```python
from build123d import *

# Parameters (mm, degrees)
BOSS_EXTRUDE1_DEPTH      = 1
SKETCH2_W                = 5
SKETCH2_H                = 4
BOSS_EXTRUDE2_DEPTH      = 1.5
CHAMFER1_SIZE            = 0.25
SKETCH4_W                = 0.5
SKETCH4_H                = 1
BOSS_EXTRUDE3_DEPTH      = 0.5
BOSS_EXTRUDE4_DEPTH      = 0.4
CHAMFER1_OF_MIRROR1_SIZE = 0.25
SKETCH6_R                = 4
BOSS_EXTRUDE5_DEPTH      = 1.5
SKETCH7_W                = 3
SKETCH7_H                = 1
BOSS_EXTRUDE6_DEPTH      = 2
BOSS_EXTRUDE7_DEPTH      = 3
CUT_EXTRUDE1_DEPTH       = 3
SKETCH10_R               = 2.5
BOSS_EXTRUDE8_DEPTH      = 0.25
CUT_EXTRUDE2_DEPTH       = 0.25
SKETCH13_R               = 2.5
BOSS_EXTRUDE11_DEPTH     = 0.25
BOSS_EXTRUDE12_START     = -0.25
SKETCH14_R               = 2.5
BOSS_EXTRUDE12_DEPTH     = 0.25
SKETCH15_R               = 3.75
BOSS_EXTRUDE13_DEPTH     = 2.5
SKETCH17_R               = 0.75
CUT_EXTRUDE3_DEPTH       = 3
CUT_EXTRUDE5_DEPTH       = 7


with BuildPart() as part:
    # Sketch1 → Boss-Extrude1 (new body)
    with BuildSketch(Plane(origin=(0, 0, 0), x_dir=(1, 0, 0), z_dir=(0, 1, 0))):
        with BuildLine():
            Line((8.75, -5), (-7.25, -5))
            ThreePointArc((-7.25, -5), (-7.689339828, -3.939339828), (-8.75, -3.5))
            Line((-8.75, -3.5), (-8.75, 3.5))
            ThreePointArc((-8.75, 3.5), (-7.689339828, 3.939339828), (-7.25, 5))
            Line((-7.25, 5), (8.75, 5))
            Line((8.75, 5), (8.75, -5))
        make_face()
    extrude(amount=BOSS_EXTRUDE1_DEPTH)

    # Sketch2 → Boss-Extrude2 (add)
    with BuildSketch(Plane(origin=(0, 1, 0), x_dir=(1, 0, 0), z_dir=(0, 1, 0))):
        with Locations((4.283897802, -1)):
            Rectangle(SKETCH2_W, SKETCH2_H)
    boss_extrude2 = extrude(amount=BOSS_EXTRUDE2_DEPTH)

    # Chamfer1
    chamfer1_edges = [part.edges().sort_by_distance(p)[0] for p in [
        (6.783897802, 2.5, 1),
        (4.283897802, 2.5, -1),
        (1.783897802, 2.5, 1),
        (4.283897802, 2.5, 3),
    ]]
    chamfer(chamfer1_edges, length=CHAMFER1_SIZE)

    # Sketch4 → Boss-Extrude3 (add)
    with BuildSketch(Plane(origin=(0, 1, 0), x_dir=(1, 0, 0), z_dir=(0, 1, 0))):
        with Locations((5.033897802, -3.5)):
            Rectangle(SKETCH4_W, SKETCH4_H)
        with Locations((6.533897802, -3.5)):
            Rectangle(SKETCH4_W, SKETCH4_H)
        with Locations((3.533897802, -3.5)):
            Rectangle(SKETCH4_W, SKETCH4_H)
        with Locations((2.033897802, -3.5)):
            Rectangle(SKETCH4_W, SKETCH4_H)
        with Locations((6.533897802, 1.5)):
            Rectangle(SKETCH4_W, SKETCH4_H)
        with Locations((5.033897802, 1.5)):
            Rectangle(SKETCH4_W, SKETCH4_H)
        with Locations((3.533897802, 1.5)):
            Rectangle(SKETCH4_W, SKETCH4_H)
        with Locations((2.033897802, 1.5)):
            Rectangle(SKETCH4_W, SKETCH4_H)
    boss_extrude3 = extrude(amount=BOSS_EXTRUDE3_DEPTH)

    # Sketch5 → Boss-Extrude4 (add)
    with BuildSketch(Plane.ZY.offset(-0.533897802)):
        Polygon((3.5, -0.622790988), (2.5, -0.622790988), (2.5, 4.75), (2.25, 5), (2.25, 11), (3.75, 11), (3.75, 5), (3.5, 4.75), align=None)
        Polygon((0.5, -0.622790988), (-0.5, -0.622790988), (-0.5, 4.75), (-0.75, 5), (-0.75, 11), (0.75, 11), (0.75, 5), (0.5, 4.75), align=None)
        Polygon((-2.5, -0.622790988), (-3.5, -0.622790988), (-3.5, 4.75), (-3.75, 5), (-3.75, 11), (-2.25, 11), (-2.25, 5), (-2.5, 4.75), align=None)
    extrude(amount=BOSS_EXTRUDE4_DEPTH)

    # Mirror1: Boss-Extrude2, Boss-Extrude3 across plane
    add(boss_extrude2.mirror(Plane.ZX.offset(0.5)))
    add(boss_extrude3.mirror(Plane.ZX.offset(0.5)))

    # Chamfer1 of Mirror1
    chamfer1_of_mirror1_edges = [part.edges().sort_by_distance(p)[0] for p in [
        (6.783897802, -1.5, 1),
        (4.283897802, -1.5, -1),
        (1.783897802, -1.5, 1),
        (4.283897802, -1.5, 3),
    ]]
    chamfer(chamfer1_of_mirror1_edges, length=CHAMFER1_OF_MIRROR1_SIZE)

    # Sketch6 → Boss-Extrude5 (add, symmetric)
    with BuildSketch(Plane(origin=(0, 11, 0), x_dir=(1, 0, 0), z_dir=(0, 1, 0))):
        with BuildLine():
            Line((0.533897802, 5), (8.533897802, 5))
            ThreePointArc((8.533897802, 5), (9.948111365, 4.414213562), (10.533897802, 3))
            Line((10.533897802, 3), (10.533897802, -3))
            ThreePointArc((10.533897802, -3), (9.948111365, -4.414213562), (8.533897802, -5))
            Line((8.533897802, -5), (0.533897802, -5))
            Line((0.533897802, -5), (0.533897802, 5))
        make_face()
        with Locations(Location((5.753897802, 0, 0), (0, 0, 270))):
            Circle(SKETCH6_R, mode=Mode.SUBTRACT)
    extrude(amount=BOSS_EXTRUDE5_DEPTH, both=True)

    # Sketch7 → Boss-Extrude6 (add)
    with BuildSketch(Plane(origin=(0, 12.5, 0), x_dir=(1, 0, 0), z_dir=(0, 1, 0))):
        with Locations((4.503897802, 4.5)):
            Rectangle(SKETCH7_W, SKETCH7_H)
    boss_extrude6 = extrude(amount=BOSS_EXTRUDE6_DEPTH)

    # Sketch8 → Boss-Extrude7 (add)
    with BuildSketch(Plane(origin=(6.003897802, 0, 0), x_dir=(0, 0, -1), z_dir=(1, 0, 0))):
        Polygon((4.5, 14.5), (5.077350269, 13.5), (4.5, 13.5), align=None)
    boss_extrude7 = extrude(amount=-BOSS_EXTRUDE7_DEPTH)

    # Sketch9 → Cut-Extrude1 (cut)
    with BuildSketch(Plane(origin=(6.003897802, 0, 0), x_dir=(0, 0, -1), z_dir=(1, 0, 0))):
        Polygon((4.5, 14.5), (5, 13.633974596), (5, 14.5), align=None)
    cut_extrude1 = extrude(amount=-CUT_EXTRUDE1_DEPTH, mode=Mode.SUBTRACT)

    # Mirror2: Boss-Extrude6, Boss-Extrude7, Cut-Extrude1 across plane
    add(boss_extrude6.mirror(Plane.XY))
    add(boss_extrude7.mirror(Plane.XY))
    add(cut_extrude1.mirror(Plane.XY), mode=Mode.SUBTRACT)

    # Sketch10 → Boss-Extrude8 (add)
    with BuildSketch(Plane.XZ.offset(-9.5)):
        with BuildLine():
            ThreePointArc((5.003897802, -3.929058411), (5.753897802, -4), (6.503897802, -3.929058411))
            Line((6.503897802, -3.929058411), (6.503897802, -3.418698583))
            ThreePointArc((6.503897802, -3.418698583), (8.228771537, -2.474873734), (9.172596385, -0.75))
            Line((9.172596385, -0.75), (9.682956214, -0.75))
            ThreePointArc((9.682956214, -0.75), (9.736122912, -0.376673834), (9.753897802, 0))
            ThreePointArc((9.753897802, 0), (9.736122912, 0.376673834), (9.682956214, 0.75))
            Line((9.682956214, 0.75), (9.172596385, 0.75))
            ThreePointArc((9.172596385, 0.75), (8.228771537, 2.474873734), (6.503897802, 3.418698583))
            Line((6.503897802, 3.418698583), (6.503897802, 3.929058411))
            ThreePointArc((6.503897802, 3.929058411), (5.753897802, 4), (5.003897802, 3.929058411))
            Line((5.003897802, 3.929058411), (5.003897802, 3.418698583))
            ThreePointArc((5.003897802, 3.418698583), (3.279024068, 2.474873734), (2.33519922, 0.75))
            Line((2.33519922, 0.75), (1.824839391, 0.75))
            ThreePointArc((1.824839391, 0.75), (1.753897802, 0), (1.824839391, -0.75))
            Line((1.824839391, -0.75), (2.33519922, -0.75))
            ThreePointArc((2.33519922, -0.75), (3.279024068, -2.474873734), (5.003897802, -3.418698583))
            Line((5.003897802, -3.418698583), (5.003897802, -3.929058411))
        make_face()
        with Locations(Location((5.753897802, 0, 0), (0, 0, 270))):
            Circle(SKETCH10_R, mode=Mode.SUBTRACT)
    extrude(amount=-BOSS_EXTRUDE8_DEPTH)

    # Sketch11 → Cut-Extrude2 (cut)
    with BuildSketch(Plane.XZ.offset(-9.5)):
        with BuildLine():
            Line((9.682956214, 0.75), (10.322596385, 0.75))
            Line((10.322596385, 0.75), (10.322596385, 3.068698583))
            ThreePointArc((10.322596385, 3.068698583), (9.883256557, 4.129358755), (8.822596385, 4.568698583))
            Line((8.822596385, 4.568698583), (6.503897802, 4.568698583))
            Line((6.503897802, 4.568698583), (6.503897802, 3.929058411))
            ThreePointArc((6.503897802, 3.929058411), (8.582324927, 2.828427125), (9.682956214, 0.75))
        make_face()
        with BuildLine():
            Line((10.322596385, -3.068698583), (10.322596385, -0.75))
            Line((10.322596385, -0.75), (9.682956214, -0.75))
            ThreePointArc((9.682956214, -0.75), (8.582324927, -2.828427125), (6.503897802, -3.929058411))
            Line((6.503897802, -3.929058411), (6.503897802, -4.568698583))
            Line((6.503897802, -4.568698583), (8.822596385, -4.568698583))
            ThreePointArc((8.822596385, -4.568698583), (9.883256557, -4.129358755), (10.322596385, -3.068698583))
        make_face()
        with BuildLine():
            Line((2.68519922, -4.568698583), (5.003897802, -4.568698583))
            Line((5.003897802, -4.568698583), (5.003897802, -3.929058411))
            ThreePointArc((5.003897802, -3.929058411), (2.925470678, -2.828427125), (1.824839391, -0.75))
            Line((1.824839391, -0.75), (1.18519922, -0.75))
            Line((1.18519922, -0.75), (1.18519922, -3.068698583))
            ThreePointArc((1.18519922, -3.068698583), (1.624539048, -4.129358755), (2.68519922, -4.568698583))
        make_face()
        with BuildLine():
            Line((1.18519922, 3.068698583), (1.18519922, 0.75))
            Line((1.18519922, 0.75), (1.824839391, 0.75))
            ThreePointArc((1.824839391, 0.75), (2.925470678, 2.828427125), (5.003897802, 3.929058411))
            Line((5.003897802, 3.929058411), (5.003897802, 4.568698583))
            Line((5.003897802, 4.568698583), (2.68519922, 4.568698583))
            ThreePointArc((2.68519922, 4.568698583), (1.624539048, 4.129358755), (1.18519922, 3.068698583))
        make_face()
    extrude(amount=-CUT_EXTRUDE2_DEPTH, mode=Mode.SUBTRACT)

    # Sketch13 → Boss-Extrude11 (add)
    with BuildSketch(Plane(origin=(0, 9.75, 0), x_dir=(1, 0, 0), z_dir=(0, 1, 0))):
        with BuildLine():
            ThreePointArc((5.753897802, -4), (9.753897802, 0), (5.753897802, 4))
            ThreePointArc((5.753897802, 4), (1.753897802, 0), (5.753897802, -4))
        make_face()
        with Locations(Location((5.753897802, 0, 0), (0, 0, 90))):
            Circle(SKETCH13_R, mode=Mode.SUBTRACT)
    extrude(amount=BOSS_EXTRUDE11_DEPTH)

    # Sketch14 → Boss-Extrude12 (add)
    with BuildSketch(Plane(origin=(0, 10, 0), x_dir=(1, 0, 0), z_dir=(0, 1, 0)).offset(BOSS_EXTRUDE12_START)):
        with Locations(Location((5.753897802, 0, 0), (0, 0, 90))):
            Circle(SKETCH14_R)
    extrude(amount=BOSS_EXTRUDE12_DEPTH)

    # Sketch15 → Boss-Extrude13 (add)
    with BuildSketch(Plane(origin=(0, 10, 0), x_dir=(1, 0, 0), z_dir=(0, 1, 0))):
        with Locations(Location((5.753897802, 0, 0), (0, 0, 90))):
            Circle(SKETCH15_R)
    extrude(amount=BOSS_EXTRUDE13_DEPTH)

    # Sketch17 → Cut-Extrude3 (cut)
    with BuildSketch(Plane(origin=(0, 12.5, 0), x_dir=(1, 0, 0), z_dir=(0, 1, 0))):
        with Locations(Location((5.753897802, 0, 0), (0, 0, 270))):
            Circle(SKETCH17_R)
    extrude(amount=-CUT_EXTRUDE3_DEPTH, mode=Mode.SUBTRACT)

    # Sketch19 → Cut-Extrude5 (cut)
    with BuildSketch(Plane(origin=(0, 12.5, 0), x_dir=(1, 0, 0), z_dir=(0, 1, 0))):
        with BuildLine():
            Line((10.533897802, -3), (10.533897802, -2.823055401))
            Line((10.533897802, -2.823055401), (8.242765452, -5))
            Line((8.242765452, -5), (8.533897802, -5))
            ThreePointArc((8.533897802, -5), (9.948111365, -4.414213562), (10.533897802, -3))
        make_face()
        with BuildLine():
            Line((8.533897802, 5), (8.242765452, 5))
            Line((8.242765452, 5), (10.533897802, 2.823055401))
            Line((10.533897802, 2.823055401), (10.533897802, 3))
            ThreePointArc((10.533897802, 3), (9.948111365, 4.414213562), (8.533897802, 5))
        make_face()
    extrude(amount=-CUT_EXTRUDE5_DEPTH, mode=Mode.SUBTRACT)


solid = part.part
```
Source: CAD feature listing. Evaluate the final solid. Frame: model axes, mm. A direction names the side the tool comes from. Coordinates: 2 decimals unless noted, no trailing zeros. Loops run counter-clockwise (first coordinate to the right, second up) from the corner with the lowest first, then second, coordinate; pieces in that order, holes last. Notation, with made-up numbers: M 49.25,82.5 L 104.25,82.5 A19 ccw 104.25,100.5 Z; hole C 69.5,-27 d8. An arc over 180 degrees is marked long. Use a Markdown table: item, result. Add a question column.
Q1. First-contact query: pin 1 (1.6 mm diameter, centred on y = 4.5, z = -2.5, fed in from -X); pin 2 (1.1 mm diameter, centred on y = 0.5, z = -1.5, fed in from +X); pin 3 (4 mm diameter, centred on x = 3.5, y = 10, fed in from +Z); pin 4 (2 mm diameter, centred on x = 6, y = 8, fed in from +Z). Flat tips, straight axial feed; report the tip coordinate or a pass-through.
Q2. Material intervals for L1, parallel to X at y = 11.7, z = 0; L2, parallel to X at y = 10.45, z = 0; L3, parallel to X at y = 9.6, z = 0, sorted ascending.
Q3. Section query C-C, the plane y = 2. Return loops of the section in (x, z).
Q4. Section query A-A, the plane y = 10.25. Return loops of the section in (x, z).
Q5. Access query for faces 1 (the flat face through (0.534, 5, 0)), 2 (the flat face through (3.004, 13.5, 4.4)), 3 (the flat face through (6, 12.5, -1)). Directions: +Z, -Z, +X, -X, +Y, -Y. A direction counts if a zero-diameter tool reaches every point of the face in a straight line with its end or side. Return the directions, or none.
Q6. Section query B-B, the plane y = 4. Return loops of the section in (x, z).
Q7. Draft query along Z for faces 4 (the flat face through (4, 2.5, 1)), 5 (the flat face through (9.4, 11, 3.9)), 6 (the cylindrical face through (2.036, 11.232, 0.488)). Return one class per face: pulls with the +Z half, pulls with the -Z half, needs draft (parallel to the pull), parting line crosses it, or undercut.
Q8. Section query D-D, the plane x = -6.5. Return loops of the section in (y, z).
Result:
| question | item | result |
|---|---|---|
| 1 | pin 1 | stops at x = 0.13 |
| 1 | pin 2 | stops at x = 8.75 |
| 1 | pin 3 | stops at z = 5 |
| 1 | pin 4 | passes through |
| 2 | L1 | x = 0.53 to 1.75, 2 to 5, 6.5 to 9.5, 9.75 to 10.53 |
| 2 | L2 | x = 0.13 to 1.75, 2 to 5, 6.5 to 9.5, 9.75 to 10.53 |
| 2 | L3 | x = 0.13 to 3.25, 8.25 to 10.53 |
| 3 | outline | M 0.13,-3.5 L 0.53,-3.5 L 0.53,-2.5 L 0.13,-2.5 Z; M 0.13,-0.5 L 0.53,-0.5 L 0.53,0.5 L 0.13,0.5 Z; M 0.13,2.5 L 0.53,2.5 L 0.53,3.5 L 0.13,3.5 Z; M 1.78,-1 L 6.78,-1 L 6.78,3 L 1.78,3 Z |
| 4 | outline | M 0.13,-3.75 L 0.53,-3.75 L 0.53,-5 L 8.24,-5 L 10.53,-2.82 L 10.53,2.82 L 8.24,5 L 0.53,5 L 0.53,3.75 L 0.13,3.75 L 0.13,2.25 L 0.53,2.25 L 0.53,0.75 L 0.13,0.75 L 0.13,-0.75 L 0.53,-0.75 L 0.53,-2.25 L 0.13,-2.25 Z; C 5.75,0 d7.5; hole C 5.75,0 d8; hole C 5.75,0 d1.5 |
| 5 | face 1 | +Z, -Z |
| 5 | face 2 | +Z, -Z, -X, +Y |
| 5 | face 3 | +X, -X, +Y |
| 6 | outline | M 0.13,-3.5 L 0.53,-3.5 L 0.53,-2.5 L 0.13,-2.5 Z; M 0.13,-0.5 L 0.53,-0.5 L 0.53,0.5 L 0.13,0.5 Z; M 0.13,2.5 L 0.53,2.5 L 0.53,3.5 L 0.13,3.5 Z |
| 7 | face 4 | needs draft |
| 7 | face 5 | pulls with the +Z half |
| 7 | face 6 | undercut |
| 8 | outline | M 0,-5 L 1,-5 L 1,5 L 0,5 Z |
